from build123d import *

# Parameters (mm, degrees)
BOX003_W     = 139
BOX003_H     = 10
BOX003_DEPTH = 10
BOX001_W     = 360
BOX001_H     = 2.5
BOX001_DEPTH = 42.5
BOX_W        = 120
BOX_H        = 37.5
BOX_DEPTH    = 2.5
BOX002_W     = 360
BOX002_H     = 27.5
BOX002_DEPTH = 2.5


with BuildPart() as cube003:
    # Box003 → Box003 (new body)
    with BuildSketch(Plane(origin=(-10, -10, -3), x_dir=(1, 0, 0), z_dir=(0, 0, 1))):
        with Locations((69.5, 5)):
            Rectangle(BOX003_W, BOX003_H)
    extrude(amount=BOX003_DEPTH)


with BuildPart() as cube001:
    # Box001 → Box001 (new body)
    with BuildSketch(Plane(origin=(-120, 0, 0), x_dir=(1, 0, 0), z_dir=(0, 0, 1))):
        with Locations((180, 1.25)):
            Rectangle(BOX001_W, BOX001_H)
    extrude(amount=BOX001_DEPTH)


with BuildPart() as fusion:
    # Box → Box (new body)
    with BuildSketch(Plane(origin=(0, -10, 0), x_dir=(1, 0, 0), z_dir=(0, 0, 1))):
        with Locations((60, 18.75)):
            Rectangle(BOX_W, BOX_H)
    extrude(amount=BOX_DEPTH)

    # Fusion: union Cube001
    add(cube001.part)


with BuildPart() as cut:
    # Box002 → Box002 (new body)
    with BuildSketch(Plane(origin=(-120, 0, 42.5), x_dir=(1, 0, 0), z_dir=(0, 0, 1))):
        with Locations((180, 13.75)):
            Rectangle(BOX002_W, BOX002_H)
    extrude(amount=BOX002_DEPTH)

    # Fusion001: union Fusion
    add(fusion.part)

    # Cut: cut Cube003
    add(cube003.part, mode=Mode.SUBTRACT)


solid = cut.part
Design review of the part built by this model. Coordinates are the model's own, in mm. A direction names the side the tool comes from. Coordinates: 2 decimals unless noted, no trailing zeros. Write each loop counter-clockwise with the first axis right and the second up, starting at its lowest first coordinate (ties: lowest second). Pieces come first, ordered by that corner, then holes. Notation, with made-up numbers: (48.25, 0) - (54.25, 0) arc R15 ccw to (54.25, 21) - close; hole circle Ø6 at (-18, 65.5). An arc over 180 degrees is marked (long way). Use one line per item in the form item = value.
Q1. Machinability: for faces 1 (the flat face through (59, 15, 2.5)), 2 (the flat face through (57, 0, 22)), which of the approach directions +Z, -Z, +X, -X, +Y, -Y give a long, thin tool a straight path to every point of the face, cutting with its end or side? Answer none if there is none.
Taken from the geometry:
face_1 = +X, -X, +Y
face_2 = +Z, -Z, +X, -X, -Y
Q2. Consider section A-A (y = 7.75). Write out the cut boundary in (x, z), plus the area to 3 significant figures.
Taken from the geometry:
outline = (-120, 42.5) - (240, 42.5) - (240, 45) - (-120, 45) - close; (0, 0) - (120, 0) - (120, 2.5) - (0, 2.5) - close
area = 1,200 mm^2
Q3. Consider section B-B (x = 5). Write out the cut boundary in (y, z), plus the area to 4 significant figures.
Taken from the geometry:
outline = (0, 0) - (27.5, 0) - (27.5, 2.5) - (2.5, 2.5) - (2.5, 42.5) - (27.5, 42.5) - (27.5, 45) - (0, 45) - close
area = 237.5 mm^2
Q4. Insertion check: pin 1 Ø3 at (y, z) = (17.5, 1) entering from -X; pin 2 Ø21 at (x, z) = (-25.5, 27.5) entering from +Y; pin 3 Ø4 at (x, y) = (187, 11.5) entering from -Z; pin 4 Ø1 at (x, z) = (-76.5, 32) entering from -Y. Each pin has a flat end and moves straight along its axis. Give the tip position at first contact, or say it passes through.
Taken from the geometry:
pin_1 = 0
pin_2 = 2.5
pin_3 = 42.5
pin_4 = 0
Q5. Consider section D-D (x = 158). Write out the cut boundary in (y, z).
Taken from the geometry:
outline = (0, 0) - (2.5, 0) - (2.5, 42.5) - (27.5, 42.5) - (27.5, 45) - (0, 45) - close
Q6. The part is to be moulded in two halves that separate along Z. For faces 3 (the flat face through (57, 15, 42.5)), 4 (the flat face through (57, 14, 45)), 5 (the flat face through (57, 11, 0)), say which applies: +Z half, -Z half, draft (parallel to the pull), parting line (faces both ways), or undercut.
Taken from the geometry:
face_3 = undercut
face_4 = +Z half
face_5 = -Z half
Q7. For probe 1 along Z at (x, y) = (65, 7); probe 2 along Z at (x, y) = (-28.5, 25.25); probe 3 along Y at (x, z) = (209, 22.5), list the stretches that pass through material, from the lowest coordinate up.
Taken from the geometry:
probe_1 = 0 to 2.5, 42.5 to 45
probe_2 = 42.5 to 45
probe_3 = 0 to 2.5
Q8. Consider section C-C (z = 7). Write out the cut boundary in (x, y).
Taken from the geometry:
outline = (-120, 0) - (240, 0) - (240, 2.5) - (-120, 2.5) - close
